from build123d import *

# Parameters (mm, degrees)
F1_DEPTH = 7


with BuildPart() as f1:
    # F0 (on Top) → F1 (new body)
    with BuildSketch(Plane.XY):
        with BuildLine():
            ThreePointArc((0, 19), (4.1112446628, 18.5498697387), (8.0276897851, 17.2208070866))
            ThreePointArc((8.0276897851, 17.2208070866), (13.5033179565, 22.8701114223), (15.5, 30.48))
            ThreePointArc((15.5, 30.48), (-7.6098885777, 43.9833179565), (-8.0276897851, 17.2208070866))
            ThreePointArc((-8.0276897851, 17.2208070866), (-4.1112446628, 18.5498697387), (0, 19))
        make_face()
        with BuildLine():
            ThreePointArc((11.025, 30.48), (7.7958522626, 22.6841477374), (0, 19.455))
            ThreePointArc((0, 19.455), (-7.7958522626, 38.2758522626), (11.025, 30.48))
        make_face(mode=Mode.SUBTRACT)
        with BuildLine():
            ThreePointArc((-9.5479300767, -5.5125), (-9.5479300767, 5.5125), (0, 11.025))
            Line((0, 11.025), (0, 14.98))
            ThreePointArc((0, 14.98), (-4.1672838782, 15.550708487), (-8.0276897851, 17.2208070866))
            ThreePointArc((-8.0276897851, 17.2208070866), (-16.4544826719, 9.5), (-18.9275013032, -1.6582202557))
            ThreePointArc((-18.9275013032, -1.6582202557), (-15.5509505357, -4.1663805402), (-12.9730605487, -7.49))
            Line((-12.9730605487, -7.49), (-9.5479300767, -5.5125))
        make_face()
        with BuildLine():
            ThreePointArc((0, 11.025), (4.6737551189, 9.985321131), (8.4660219047, 7.0623719889))
            Line((8.4660219047, 7.0623719889), (18.9753399185, 0.9677163728))
            ThreePointArc((18.9753399185, 0.9677163728), (15.7585418973, 10.6145351886), (8.0276897851, 17.2208070866))
            ThreePointArc((8.0276897851, 17.2208070866), (4.1672838782, 15.550708487), (0, 14.98))
            Line((0, 14.98), (0, 11.025))
        make_face()
        with BuildLine():
            ThreePointArc((-8.0276897851, 17.2208070866), (-4.1672838782, 15.550708487), (0, 14.98))
            Line((0, 14.98), (0, 19))
            ThreePointArc((0, 19), (-4.1112446628, 18.5498697387), (-8.0276897851, 17.2208070866))
        make_face()
        with BuildLine():
            Line((0, 19), (0, 14.98))
            ThreePointArc((0, 14.98), (4.1672838782, 15.550708487), (8.0276897851, 17.2208070866))
            ThreePointArc((8.0276897851, 17.2208070866), (4.1112446628, 18.5498697387), (0, 19))
        make_face()
        with BuildLine():
            ThreePointArc((-10.8998115181, -15.5625868309), (-14.0090360992, -12.8353771885), (-16.4544826719, -9.5))
            ThreePointArc((-16.4544826719, -9.5), (-18.120280762, -5.7144925502), (-18.9275013032, -1.6582202557))
            ThreePointArc((-18.9275013032, -1.6582202557), (-39.819848066, -22.99), (-10.8998115181, -15.5625868309))
        make_face()
        with BuildLine():
            ThreePointArc((-15.3714543073, -15.24), (-37.0457865422, -18.0934799723), (-16.8485242306, -9.7275))
            ThreePointArc((-16.8485242306, -9.7275), (-15.7471220725, -12.3865200277), (-15.3714543073, -15.24))
        make_face(mode=Mode.SUBTRACT)
        with BuildLine():
            Line((-16.4544826719, -9.5), (-12.9730605487, -7.49))
            ThreePointArc((-12.9730605487, -7.49), (-15.5509505357, -4.1663805402), (-18.9275013032, -1.6582202557))
            ThreePointArc((-18.9275013032, -1.6582202557), (-18.120280762, -5.7144925502), (-16.4544826719, -9.5))
        make_face()
        with BuildLine():
            ThreePointArc((-10.8964543073, -15.24), (-11.4246039999, -11.2283048009), (-12.9730605487, -7.49))
            Line((-12.9730605487, -7.49), (-16.4544826719, -9.5))
            ThreePointArc((-16.4544826719, -9.5), (-14.0090360992, -12.8353771885), (-10.8998115181, -15.5625868309))
            ThreePointArc((-10.8998115181, -15.5625868309), (-10.8972936328, -15.40130215), (-10.8964543073, -15.24))
        make_face()
        with BuildLine():
            Line((12.9730605487, -7.49), (9.5479300767, -5.5125))
            ThreePointArc((9.5479300767, -5.5125), (0, -11.025), (-9.5479300767, -5.5125))
            Line((-9.5479300767, -5.5125), (-12.9730605487, -7.49))
            ThreePointArc((-12.9730605487, -7.49), (-11.4246039999, -11.2283048009), (-10.8964543073, -15.24))
            ThreePointArc((-10.8964543073, -15.24), (-10.8972936328, -15.40130215), (-10.8998115181, -15.5625868309))
            ThreePointArc((-10.8998115181, -15.5625868309), (0, -19), (10.8998115181, -15.5625868309))
            ThreePointArc((10.8998115181, -15.5625868309), (11.3836666575, -11.3843279468), (12.9730605487, -7.49))
        make_face()
        with BuildLine():
            Line((16.4544826719, -9.5), (12.9730605487, -7.49))
            ThreePointArc((12.9730605487, -7.49), (11.3836666575, -11.3843279468), (10.8998115181, -15.5625868309))
            ThreePointArc((10.8998115181, -15.5625868309), (14.0090360992, -12.8353771885), (16.4544826719, -9.5))
        make_face()
        with BuildLine():
            ThreePointArc((8.4660219047, 7.0623719889), (10.3655322222, 3.7558443459), (11.025, 0))
            ThreePointArc((11.025, 0), (10.6493322348, -2.8534799723), (9.5479300767, -5.5125))
            Line((9.5479300767, -5.5125), (12.9730605487, -7.49))
            ThreePointArc((12.9730605487, -7.49), (15.5509505357, -4.1663805402), (18.9275013032, -1.6582202557))
            ThreePointArc((18.9275013032, -1.6582202557), (18.9818666727, -0.8299021746), (19, 0))
            ThreePointArc((19, 0), (18.9938339791, 0.4840152626), (18.9753399185, 0.9677163728))
            Line((18.9753399185, 0.9677163728), (8.4660219047, 7.0623719889))
        make_face()
        with BuildLine():
            ThreePointArc((18.9275013032, -1.6582202557), (15.5509505357, -4.1663805402), (12.9730605487, -7.49))
            Line((12.9730605487, -7.49), (16.4544826719, -9.5))
            ThreePointArc((16.4544826719, -9.5), (18.120280762, -5.7144925502), (18.9275013032, -1.6582202557))
        make_face()
        with BuildLine():
            ThreePointArc((18.9275013032, -1.6582202557), (18.120280762, -5.7144925502), (16.4544826719, -9.5))
            ThreePointArc((16.4544826719, -9.5), (14.0090360992, -12.8353771885), (10.8998115181, -15.5625868309))
            ThreePointArc((10.8998115181, -15.5625868309), (26.5577564573, -30.7391606746), (41.8964543073, -15.24))
            ThreePointArc((41.8964543073, -15.24), (34.2857264042, -1.8979841935), (18.9275013032, -1.6582202557))
        make_face()
        with BuildLine():
            ThreePointArc((37.4214543073, -15.24), (23.5429743351, -25.8893322348), (16.8485242306, -9.7275))
            ThreePointArc((16.8485242306, -9.7275), (29.2499342796, -4.5906677652), (37.4214543073, -15.24))
        make_face(mode=Mode.SUBTRACT)
    extrude(amount=F1_DEPTH)


solid = f1.part
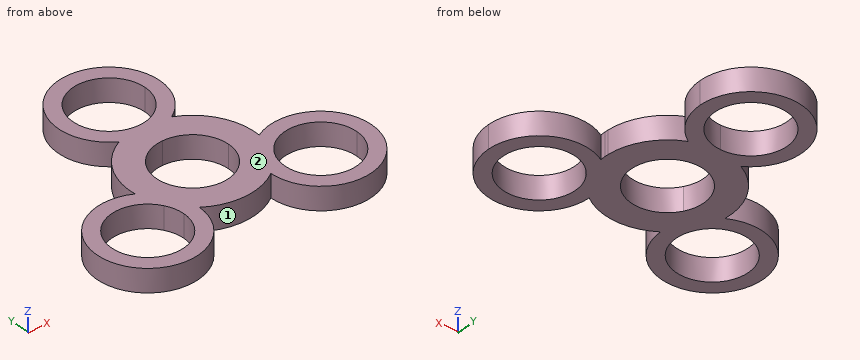
Build history of the part. All positions in model axes, mm. Face numbers are marked on the shaded views. Round coordinates to 2 decimals unless told otherwise and drop trailing zeros. Write each loop counter-clockwise with the first axis right and the second up, starting at its lowest first coordinate (ties: lowest second). Pieces come first, ordered by that corner, then holes. Notation, with made-up numbers: M -7.5,28.5 L 7.5,28.5 A17 cw 7.5,42.5 Z; hole C 6,-4.75 d9. An arc over 180 degrees is marked long. Answer in a Markdown table with one row per item.
1. Mould opens along X. For the marked faces 1 and 2 say: +X half, -X half, draft (parallel to the pull), parting line (faces both ways), or undercut.
Geometry check:
| item | result |
|---|---|
| face 1 | undercut |
| face 2 | draft |
2. Saw through at D-D (z = 2). State how many separate pieces and enclosed holes the cut face has, and give its area (3 significant figures).
Geometry check:
| item | result |
|---|---|
| separate pieces | 1 |
| enclosed holes | 4 |
| area | 1,740 mm2 |
3. Saw through at B-B (y = -12). List the corners of the cut face in (x, z), and give its area (3 significant figures).
Geometry check:
| item | result |
|---|---|
| outline | M -41.55,0 L -36.93,0 L -36.93,7 L -41.55,7 Z; M -15.86,0 L 15.86,0 L 15.86,7 L -15.86,7 Z; M 36.93,0 L 41.55,0 L 41.55,7 L 36.93,7 Z |
| area | 287 mm2 |
4. Saw through at A-A (x = -20). List the corners of the cut face in (y, z), and give its area (3 significant figures).
Geometry check:
| item | result |
|---|---|
| outline | M -29.36,0 L -24.22,0 L -24.22,7 L -29.36,7 Z; M -6.26,0 L -1.12,0 L -1.12,7 L -6.26,7 Z |
| area | 71.9 mm2 |
5. Saw through at C-C (x = 3). List the corners of the cut face in (y, z).
Geometry check:
| item | result |
|---|---|
| outline | M -18.76,0 L -10.61,0 L -10.61,7 L -18.76,7 Z; M 10.61,0 L 19.87,0 L 19.87,7 L 10.61,7 Z; M 41.09,0 L 45.69,0 L 45.69,7 L 41.09,7 Z |
6. Flat gauge pins, fed straight in: P1, Ø20, axis at x = -26.4, y = -15.24, coming from the -Z side; P2, Ø1.5, axis at x = -5, z = 3.5, coming from the +Y side; P3, Ø2, axis at y = -23, z = 6, coming from the +X side; P4, Ø2, axis at y = -7, z = 5.5, coming from the -X side. Where does each tip first touch, or does it go through?
Geometry check:
| item | result |
|---|---|
| P1 | through |
| P2 | y = 45.39 |
| P3 | x = 40.34 |
| P4 | x = -40.1 |
7. Probe L1, parallel to X at y = 30.48, z = 1.5 (3 decimals); L2, parallel to Y at x = 26.5, z = 4.5; L3, parallel to Y at x = -10, z = 5. List the from-to ranges inside material, lowest first. Write a range as [from, to].
Geometry check:
| item | result |
|---|---|
| L1 | [-15.5, -11.025], [11.025, 15.5] |
| L2 | [-30.74, -26.26], [-4.22, 0.26] |
| L3 | [-16.16, -4.64], [4.64, 16.16], [18.64, 25.84], [35.12, 42.32] |
